Study the drawing (mm; zero at the part's minimum x, y, z) and answer. A direction names the side the tool comes from. Coordinates: 2 decimals unless noted, no trailing zeros. Order: outer loops, then holes, each group sorted by start corner. A loop starts at its lowest first (then second) coordinate and runs counter-clockwise, first axis right, second up. Notation, with made-up numbers: M 16,36.5 L 70,36.5 A9 cw 70,42.5 Z; hole C 33,40 d10. An arc over 180 degrees is marked long. Use a Markdown table: item, result. Add a question column.
1) Find the intervals of material crossed by probe 1 along X at (y, z) = (6.75, 30.5); probe 2 along X at (y, z) = (5.75, 6.5); probe 3 along Z at (x, y) = (25, 9), in increasing order. Write a range as [from, to].
2) Find section B-B on x = 21. Write down the section's boundary in (y, z).
3) Find section C-C on y = 4.5. Write down the section's boundary in (x, z).
4) For the marked faces 1, 2 and 3, determine the directions among +Z, -Z, +X, -X, +Y, -Y from which every point of the face is accessible in a straight line to the end or side of a thin tool.
5) Each of these flat-tipped pins is pushed along its axis until it touches: pin 1 Ø2 at (x, y) = (10, 8) entering from +Z; pin 2 Ø2 at (y, z) = (1.5, 4) entering from -X. Where does it stop, or does it pass through?
6) Find section A-A on z = 17. Write down the section's boundary in (x, y).
7) Find section D-D on z = 25.5. Write down the section's boundary in (x, y).
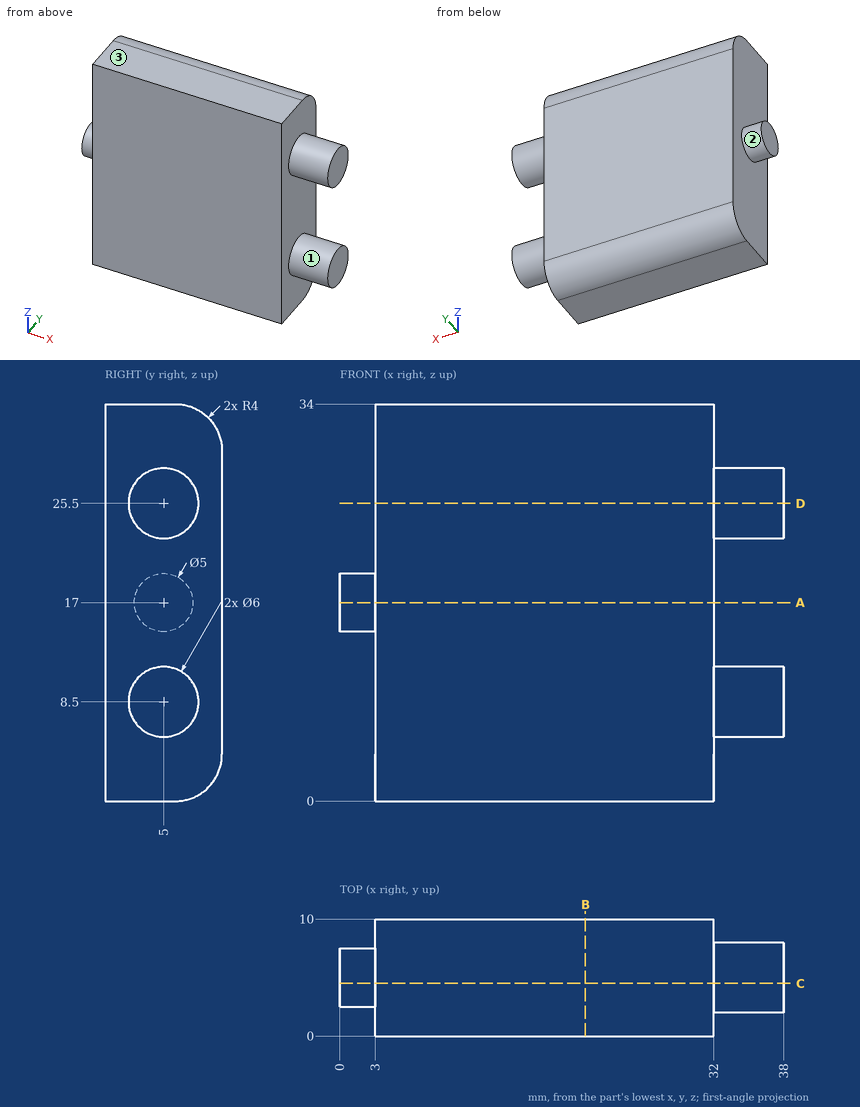
Check result:
| question | item | result |
|---|---|---|
| 1 | probe 1 | x = [3, 32] |
| 1 | probe 2 | x = [3, 38] |
| 1 | probe 3 | z = [1.35, 32.65] |
| 2 | outline | M 0,0 L 6,0 A4 ccw 10,4 L 10,30 A4 ccw 6,34 L 0,34 Z |
| 3 | outline | M 0,14.55 L 3,14.55 L 3,0 L 32,0 L 32,5.54 L 38,5.54 L 38,11.46 L 32,11.46 L 32,22.54 L 38,22.54 L 38,28.46 L 32,28.46 L 32,34 L 3,34 L 3,19.45 L 0,19.45 Z |
| 4 | face 1 | +X |
| 4 | face 2 | -X |
| 4 | face 3 | +Z, +X, -X, +Y, -Y |
| 5 | pin 1 | stops at z = 33.87 |
| 5 | pin 2 | stops at x = 3 |
| 6 | outline | M 0,2.5 L 3,2.5 L 3,0 L 32,0 L 32,10 L 3,10 L 3,7.5 L 0,7.5 Z |
| 7 | outline | M 3,0 L 32,0 L 32,2 L 38,2 L 38,8 L 32,8 L 32,10 L 3,10 Z |
